Geometry check sheet. Reference: the model listing, model coordinates, mm. A direction names the side the tool comes from. Round coordinates to 2 decimals unless told otherwise and drop trailing zeros. Loops run counter-clockwise (first coordinate to the right, second up) from the corner with the lowest first, then second, coordinate; pieces in that order, holes last. Notation, with made-up numbers: (79.5, 28.5) - (85.5, 28.5) arc R16 ccw to (85.5, 59.5) - close; hole circle Ø1 at (-36, 56.25). An arc over 180 degrees is marked (long way). Answer as CSV lines item,"result". Start each with the question number.
1) Draft check along Y on faces 1 (the flat face through (68, -1, 41)), 2 (the cylindrical face through (-81, 0, 1)), 3 (the flat face through (-1, -68, 41)). Enter one of: released by +Y, released by -Y, zero draft, split by the parting line, or undercut.
2) Cross-section at C-C on z = 48. Record the boundary of the cut face in (x, y).
3) Thickness scan on line 1 along Y through (x, z) = (0, 0.6); line 2 along X through (y, z) = (-62, 25). Record the ranges inside material, lowest first.
4) Cross-section at B-B on y = 28. Record the boundary of the cut face in (x, z), and give its area (3 significant figures).
5) Cross-section at D-D on x = 0. Record the boundary of the cut face in (y, z), and give its area (3 significant figures).
6) Access from +Z, -Z, +X, -X, +Y, -Y to the whole of each face (thin tool, end or side, straight path). Record for faces 4 (the flat face through (-68, -1, 41)), 5 (the flat face through (-1, 68, 41)), 6 (the flat face through (-65, -1, 39)), 7 (the cylindrical face through (80.66, -1.72, 1.01)).
7) Depth check by flat-ended pin: P1, Ø1, axis at y = -19.5, z = 71.5, coming from the +X side; P2, Ø2, axis at y = -63.5, z = 22.5, coming from the -X side; P3, Ø12, axis at x = -19.5, y = -23.5, coming from the -Z side; P4, Ø8, axis at x = 0, y = 76.5, coming from the -Z side. Enter the tip coordinate at first touch or a pass-through.
8) Cross-section at A-A on x = 76.5. Record the boundary of the cut face in (y, z).
from build123d import *

# Parameters (mm, degrees)
F0_W     = 170
F0_H     = 170
F0_W_2   = 130
F0_H_2   = 130
F1_DEPTH = 2
F2_W     = 136
F2_H     = 136
F3_DEPTH = 80
F4_W     = 130
F4_H     = 130
F5_DEPTH = 77
F6_R     = 35
F7_DEPTH = 82.001
F8_R     = 4.5
F9_DEPTH = 2.001


with BuildPart() as f1:
    # F0 (on Top) → F1 (new body)
    with BuildSketch(Plane.XY):
        Rectangle(F0_W, F0_H)
        Rectangle(F0_W_2, F0_H_2, mode=Mode.SUBTRACT)
    extrude(amount=F1_DEPTH)

    # F2 (on face) → F3 (join)
    with BuildSketch(Plane.XY.offset(2)):
        Rectangle(F2_W, F2_H)
    extrude(amount=F3_DEPTH)

    # F4 (on face) → F5 (cut)
    with BuildSketch(Plane(origin=(0, 0, 2), x_dir=(1, 0, 0), z_dir=(0, 0, -1))):
        Rectangle(F4_W, F4_H)
    extrude(amount=-F5_DEPTH, mode=Mode.SUBTRACT)

    # F6 (on face) → F7 (cut, through all)
    with BuildSketch(Plane.XY.offset(82)):
        Circle(F6_R)
    extrude(amount=-F7_DEPTH, mode=Mode.SUBTRACT)

    # F8 (on face) → F9 (cut, through all)
    with BuildSketch(Plane.XY.offset(2)):
        with Locations((0, 76.5)):
            Circle(F8_R)
        with Locations((-76.5, 0)):
            Circle(F8_R)
        with Locations((76.5, 0)):
            Circle(F8_R)
        with Locations((0, -76.5)):
            Circle(F8_R)
    extrude(amount=-F9_DEPTH, mode=Mode.SUBTRACT)


solid = f1.part
Answer block:
1,face 1,"zero draft"
1,face 2,"undercut"
1,face 3,"released by -Y"
2,outline,"(-68, -68) - (68, -68) - (68, 68) - (-68, 68) - close; hole (-65, -65) - (65, -65) - (65, 65) - (-65, 65) - close"
3,line 1,"y = -85 to -81, -72 to -65, 65 to 72, 81 to 85"
3,line 2,"x = -68 to -65, 65 to 68"
4,outline,"(-85, 0) - (-65, 0) - (-65, 79) - (-21, 79) - (-21, 82) - (-68, 82) - (-68, 2) - (-85, 2) - close; (21, 79) - (65, 79) - (65, 0) - (85, 0) - (85, 2) - (68, 2) - (68, 82) - (21, 82) - close"
4,area,"824 mm^2"
5,outline,"(-85, 0) - (-81, 0) - (-81, 2) - (-85, 2) - close; (-72, 0) - (-65, 0) - (-65, 79) - (-35, 79) - (-35, 82) - (-68, 82) - (-68, 2) - (-72, 2) - close; (35, 79) - (65, 79) - (65, 0) - (72, 0) - (72, 2) - (68, 2) - (68, 82) - (35, 82) - close; (81, 0) - (85, 0) - (85, 2) - (81, 2) - close"
5,area,"704 mm^2"
6,face 4,"+Z, -X, +Y, -Y"
6,face 5,"+Z, +X, -X, +Y"
6,face 6,"-Z"
6,face 7,"+Z, -Z"
7,P1,"stops at x = 68"
7,P2,"stops at x = -68"
7,P3,"stops at z = 79"
7,P4,"passes through"
8,outline,"(-85, 0) - (-4.5, 0) - (-4.5, 2) - (-85, 2) - close; (4.5, 0) - (85, 0) - (85, 2) - (4.5, 2) - close"
